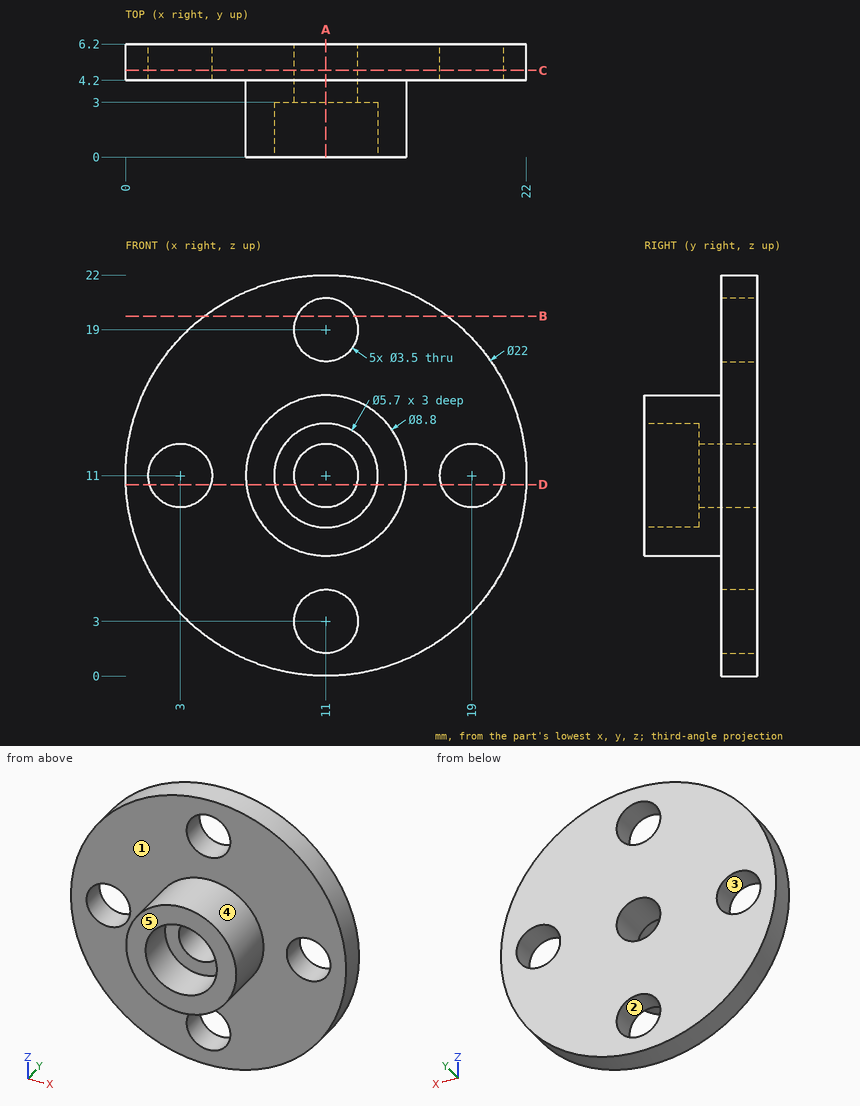
Print and shaded views of the part. All mm, measured from the part's lowest x, y and z. A direction names the side the tool comes from. Give positions to 0.01 mm unless a question says otherwise; leave off trailing zeros. Loops run counter-clockwise (first coordinate to the right, second up) from the corner with the lowest first, then second, coordinate; pieces in that order, holes last. Notation, with made-up numbers: (33.5, 59.25) -> (83.5, 59.25) arc R23 ccw to (83.5, 89.25) -> close; hole circle Ø5 at (-33.5, 39.5). An arc over 180 degrees is marked (long way). One line per question, with ' | ' between items. Start each with the question number.
1) Pin check, flat tips, straight feed: pin 1 (1.7 mm diameter, centred on x = 9.5, z = 12, fed in from -Y); pin 2 (1 mm diameter, centred on x = 9.5, z = 4.5, fed in from -Y); pin 3 (3 mm diameter, centred on x = 11, z = 11, fed in from -Y). Stop position of each tip, or through.
2) Probe L1, parallel to Z at x = 11, y = 5.75; L2, parallel to Z at x = 11, y = 2.1. List the from-to ranges inside material, lowest first.
3) Cut at C-C (y = 4.75). Give the cut face in (x, z), plus the area to 3 significant figures.
4) Two-plate mould, pull along X, no slides. Class the marked faces 3, 4 and 5: released by +X, released by -X, zero draft, split by the parting line, or undercut.
5) Cut at B-B (z = 19.75). Give the cut face in (x, y), plus the area to 3 significant figures.
6) Cut at D-D (z = 10.5). Give the cut face in (x, y), plus the area to 3 significant figures.
7) 3-axis set-ups, long thin cutter, end or side, ignore diameter. For the marked faces 1 and 2: which of +Z, -Z, +X, -X, +Y, -Y reach the whole face in a straight line?
8) Cut at A-A (x = 11). Give the cut face in (y, z), plus the area to 3 significant figures.
Return value:
1) pin 1: y = 3 | pin 2: y = 4.2 | pin 3: through
2) L1: 0 to 1.25, 4.75 to 9.25, 12.75 to 17.25, 20.75 to 22 | L2: 6.6 to 8.15, 13.85 to 15.4
3) outline: circle Ø22 at (11, 11); hole circle Ø3.5 at (3, 11); hole circle Ø3.5 at (11, 3); hole circle Ø3.5 at (11, 11); hole circle Ø3.5 at (11, 19); hole circle Ø3.5 at (19, 11) | area: 332 mm^2
4) face 3: undercut | face 4: split by the parting line | face 5: zero draft
5) outline: (4.33, 4.2) -> (9.42, 4.2) -> (9.42, 6.2) -> (4.33, 6.2) -> close; (12.58, 4.2) -> (17.67, 4.2) -> (17.67, 6.2) -> (12.58, 6.2) -> close | area: 20.3 mm^2
6) outline: (0.01, 4.2) -> (1.32, 4.2) -> (1.32, 6.2) -> (0.01, 6.2) -> close; (4.68, 4.2) -> (6.63, 4.2) -> (6.63, 0) -> (8.19, 0) -> (8.19, 3) -> (9.32, 3) -> (9.32, 6.2) -> (4.68, 6.2) -> close; (12.68, 3) -> (13.81, 3) -> (13.81, 0) -> (15.37, 0) -> (15.37, 4.2) -> (17.32, 4.2) -> (17.32, 6.2) -> (12.68, 6.2) -> close; (20.68, 4.2) -> (21.99, 4.2) -> (21.99, 6.2) -> (20.68, 6.2) -> close | area: 39.7 mm^2
7) face 1: -Y | face 2: +Y, -Y
8) outline: (0, 6.6) -> (4.2, 6.6) -> (4.2, 4.75) -> (6.2, 4.75) -> (6.2, 9.25) -> (3, 9.25) -> (3, 8.15) -> (0, 8.15) -> close; (0, 13.85) -> (3, 13.85) -> (3, 12.75) -> (6.2, 12.75) -> (6.2, 17.25) -> (4.2, 17.25) -> (4.2, 15.4) -> (0, 15.4) -> close; (4.2, 0) -> (6.2, 0) -> (6.2, 1.25) -> (4.2, 1.25) -> close; (4.2, 20.75) -> (6.2, 20.75) -> (6.2, 22) -> (4.2, 22) -> close | area: 38.7 mm^2
